Design review of the part shown in the three views and the two pictorial views. Dimensions are in mm from the part's minimum x, y and z. A direction names the side the tool comes from. Give positions to 0.01 mm unless a question says otherwise; leave off trailing zeros. Loops run counter-clockwise (first coordinate to the right, second up) from the corner with the lowest first, then second, coordinate; pieces in that order, holes last. Notation, with made-up numbers: (86, 60.25) -> (110, 60.25) arc R20 cw to (110, 86.25) -> close; hole circle Ø1 at (15.25, -3). An arc over 180 degrees is marked (long way). Answer as CSV lines item,"result". Start each with the question number.
Item 1: Clearance check with a flat-ended pin moving along its axis: P1, Ø6, axis at y = 69, z = 23, coming from the +X side. State where the tip first meets the part, or that it passes through.
Item 2: Add section B-B on z = 25. State the section outline as (x, y) points.
Item 3: Machinability: for the marked faces 1 and 2, which of the approach directions +Z, -Z, +X, -X, +Y, -Y give a long, thin tool a straight path to every point of the face, cutting with its end or side? Answer none if there is none.
Item 4: For L1, parallel to Y at x = 59, z = 39.5; L2, parallel to X at y = 17, z = 30; L3, parallel to Z at x = 26, y = 19, list the stretches that pass through material, from the lowest coordinate up. Write a range as from..to.
Item 5: Add section C-C on y = 43. State the section outline as (x, z) points.
Item 6: Add section D-D on x = 54. State the section outline as (y, z) points.
Item 7: Add section A-A on x = 25. State the section outline as (y, z) points.
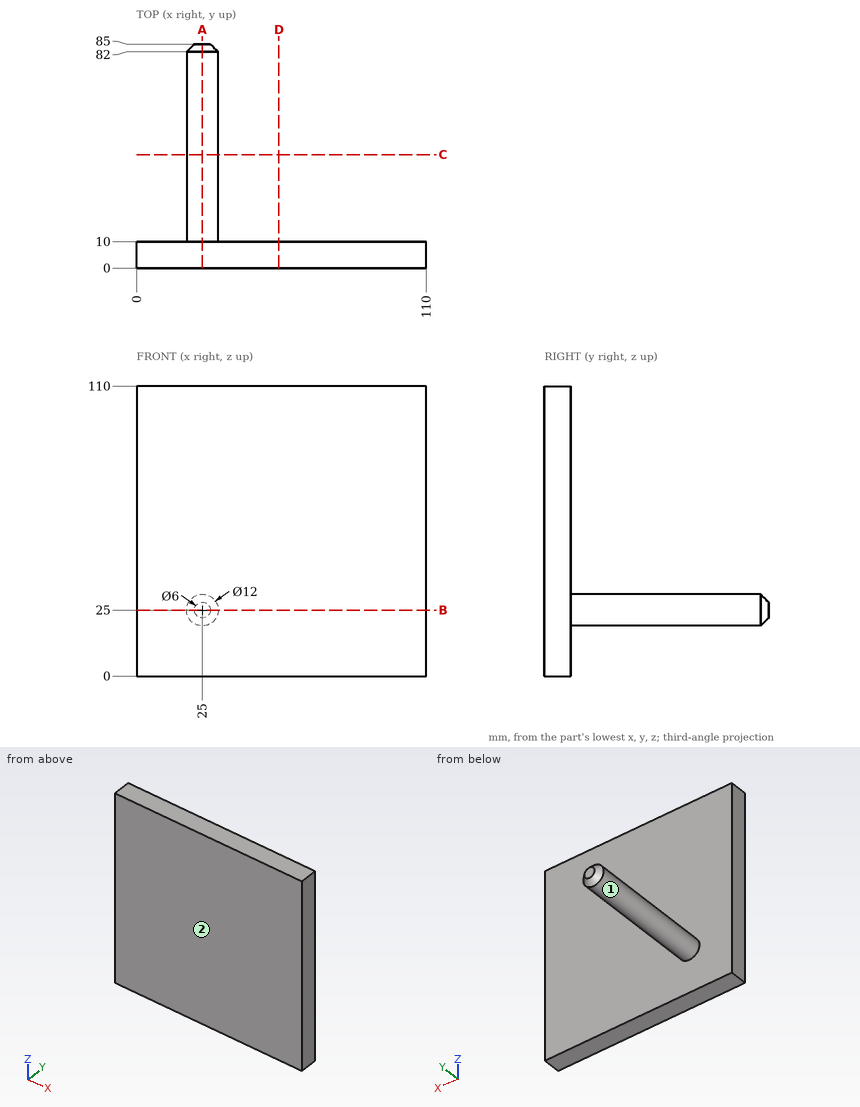
Computed values:
1,P1,"x = 31"
2,outline,"(0, 0) -> (110, 0) -> (110, 10) -> (31, 10) -> (31, 82) -> (28, 85) -> (22, 85) -> (19, 82) -> (19, 10) -> (0, 10) -> close"
3,face 1,"+Y"
3,face 2,"+Z, -Z, +X, -X, -Y"
4,L1,"0..10"
4,L2,"21.68..28.32"
4,L3,"19.08..30.92"
5,outline,"circle Ø12 at (25, 25)"
6,outline,"(0, 0) -> (10, 0) -> (10, 110) -> (0, 110) -> close"
7,outline,"(0, 0) -> (10, 0) -> (10, 19) -> (82, 19) -> (85, 22) -> (85, 28) -> (82, 31) -> (10, 31) -> (10, 110) -> (0, 110) -> close"
